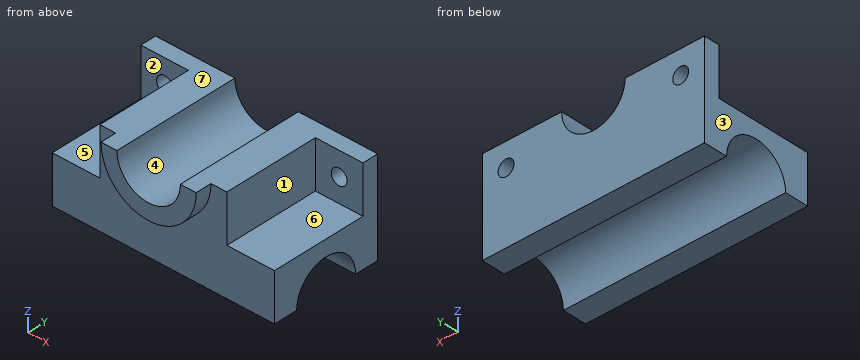
```python
from build123d import *

# Parameters (mm, degrees)
F0_W      = 140
F0_H      = 70
F1_DEPTH  = 60
F2_W      = 30
F2_H      = 30
F3_DEPTH  = 60
F4_DEPTH  = 60
F5_R      = 5
F6_DEPTH  = 10
F8_DEPTH  = 70
F10_DEPTH = 140
F11_DEPTH = 10


with BuildPart() as f1:
    # F0 (on Top) → F1 (new body)
    with BuildSketch(Plane.XY):
        with Locations((70, 35)):
            Rectangle(F0_W, F0_H)
    extrude(amount=F1_DEPTH)

    # F2 (on face) → F3 (cut)
    with BuildSketch(Plane.XZ):
        with Locations((15, 45)):
            Rectangle(F2_W, F2_H)
    extrude(amount=-F3_DEPTH, mode=Mode.SUBTRACT)

    # F2 (on face) → F4 (cut)
    with BuildSketch(Plane.XZ):
        with Locations((125, 45)):
            Rectangle(F2_W, F2_H)
    extrude(amount=-F4_DEPTH, mode=Mode.SUBTRACT)

    # F5 (on face) → F6 (cut, through all)
    with BuildSketch(Plane.XZ.offset(-60)):
        with Locations((15, 45)):
            Circle(F5_R)
        with Locations((125, 45)):
            Circle(F5_R)
    extrude(amount=-F6_DEPTH, mode=Mode.SUBTRACT)

    # F7 (on face) → F8 (cut, through all)
    with BuildSketch(Plane.XZ):
        with BuildLine():
            ThreePointArc((50, 60), (70, 40), (90, 60))
            Line((90, 60), (50, 60))
        make_face()
    extrude(amount=-F8_DEPTH, mode=Mode.SUBTRACT)

    # F9 (on face) → F10 (cut, through all)
    with BuildSketch(Plane.YZ.offset(140)):
        with BuildLine():
            Line((15, 0), (55, 0))
            ThreePointArc((55, 0), (35, 20), (15, 0))
        make_face()
    extrude(amount=-F10_DEPTH, mode=Mode.SUBTRACT)

    # F7 (on face) → F11 (join)
    with BuildSketch(Plane.XZ):
        with BuildLine():
            Line((100, 60), (90, 60))
            ThreePointArc((90, 60), (70, 40), (50, 60))
            Line((50, 60), (40, 60))
            ThreePointArc((40, 60), (70, 30), (100, 60))
        make_face()
    extrude(amount=F11_DEPTH)


solid = f1.part
```
For this review, take the finished solid that the model builds, in its own axes (mm). Face numbers are marked on the shaded views. A direction names the side the tool comes from. Round coordinates to 2 decimals unless told otherwise and drop trailing zeros. Write each loop counter-clockwise with the first axis right and the second up, starting at its lowest first coordinate (ties: lowest second). Pieces come first, ordered by that corner, then holes. Notation, with made-up numbers: M -0.5,71 L 44.5,71 A34 ccw 44.5,101 Z; hole C 31,78 d4. An arc over 180 degrees is marked long. One line per item, written item: value. Start each with the question number.
(1) We need section A-A (x = 125). Give the boundary of the cut face in (y, z).
(2) Wall thickness on line 1 (Z direction, x = 125, y = 64.25); line 2 (Y direction, x = 11.5, z = 32); line 3 (Y direction, x = 91, z = 28): over which ranges is each line inside the solid? List them lowest first.
(3) Insertion check: pin 1 (15 mm diameter, centred on x = 22, y = 33.5, fed in from +Z); pin 2 (16 mm diameter, centred on x = 15, z = 45, fed in from -Y); pin 3 (12 mm diameter, centred on x = 86, z = 31.5, fed in from -Y); pin 4 (5 mm diameter, centred on y = 55.5, z = 37.5, fed in from +X). Each pin has a flat end and moves straight along its axis. Give the tip position at first contact, or say it passes through.
(4) The part is to be moulded in two halves that separate along X. For the marked faces 1, 2, 3 and 4, say which applies: released by +X, released by -X, zero draft, split by the parting line, or undercut.
(5) Machinability: for the marked faces 5, 6 and 7, which of the approach directions +Z, -Z, +X, -X, +Y, -Y give a long, thin tool a straight path to every point of the face, cutting with its end or side? Answer none if there is none.
(6) We need section D-D (z = 41.5). Give the boundary of the cut face in (x, y).
(7) We need section C-C (x = 70). Give the boundary of the cut face in (y, z).
(8) We need section B-B (y = 35). Give the boundary of the cut face in (x, z).
Result:
1. outline: M 0,0 L 15,0 A20 cw 55,0 L 70,0 L 70,40 L 60,40 L 60,30 L 0,30 Z; M 60,50 L 70,50 L 70,60 L 60,60 Z
2. line 1: 0 to 40, 50 to 60
2. line 2: 60 to 70
2. line 3: 0 to 70
3. pin 1: z = 30
3. pin 2: y = 60
3. pin 3: y = -10
3. pin 4: x = 110
4. face 1: released by +X
4. face 2: zero draft
4. face 3: released by -X
4. face 4: undercut
5. face 5: +Z, -X, -Y
5. face 6: +Z, +X, -Y
5. face 7: +Z, +X, -X, +Y, -Y
6. outline: M 0,60 L 11.43,60 L 11.43,70 L 0,70 Z; M 18.57,60 L 30,60 L 30,0 L 46.38,0 L 46.38,-10 L 62.4,-10 L 62.4,70 L 18.57,70 Z; M 77.6,-10 L 93.62,-10 L 93.62,0 L 110,0 L 110,60 L 121.43,60 L 121.43,70 L 77.6,70 Z; M 128.57,60 L 140,60 L 140,70 L 128.57,70 Z
7. outline: M -10,30 L 0,30 L 0,0 L 15,0 A20 cw 55,0 L 70,0 L 70,40 L -10,40 Z
8. outline: M 0,20 L 140,20 L 140,30 L 110,30 L 110,60 L 90,60 A20 cw 50,60 L 30,60 L 30,30 L 0,30 Z
